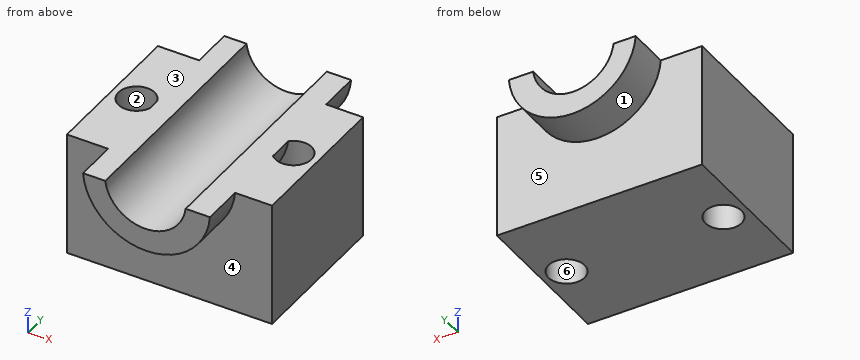
```python
from build123d import *

# Parameters (mm, degrees)
F0_W     = 86.4731967449
F0_H     = 64.1862973571
F1_DEPTH = 52.578
F2_R     = 7.62
F3_DEPTH = 180.34
F5_DEPTH = 49.784
F7_DEPTH = 69.342


with BuildPart() as f1:
    # F0 (on Top) → F1 (new body)
    with BuildSketch(Plane.XY):
        Rectangle(F0_W, F0_H)
    extrude(amount=F1_DEPTH)

    # F2 (on Top) → F3 (cut)
    with BuildSketch(Plane.XY):
        with Locations((33.0765983725, 0)):
            Circle(F2_R)
        with Locations((-33.0765983725, 0)):
            Circle(F2_R)
    extrude(amount=F3_DEPTH, mode=Mode.SUBTRACT)

    # F4 (on Front) → F5 (join, symmetric)
    with BuildSketch(Plane.XZ):
        with BuildLine():
            ThreePointArc((17.383787781, 52.578), (0.4457375035, 37.4617067344), (-16.4923127741, 52.578))
            Line((-16.4923127741, 52.578), (-25.8528143167, 52.578))
            ThreePointArc((-25.8528143167, 52.578), (0.8914759383, 27.7956383617), (27.6357661933, 52.578))
            Line((27.6357661933, 52.578), (17.383787781, 52.578))
        make_face()
    extrude(amount=F5_DEPTH, both=True)

    # F7 (cut): a face of the model
    f7_faces = [f1.faces().sort_by_distance(p)[0] for p in [
        (0.4457375035, 32.0931486785, 46.2197735841),
    ]]
    extrude(f7_faces, amount=-F7_DEPTH, mode=Mode.SUBTRACT)


solid = f1.part
```
The model under review builds one solid part; all positions refer to its coordinate system, in mm. Face numbers are marked on the shaded views. A direction names the side the tool comes from. Give positions to 0.01 mm unless a question says otherwise; leave off trailing zeros. Write each loop counter-clockwise with the first axis right and the second up, starting at its lowest first coordinate (ties: lowest second). Pieces come first, ordered by that corner, then holes. Notation, with made-up numbers: (17, 54.25) -> (59, 54.25) arc R22 ccw to (59, 90.25) -> close; hole circle Ø8 at (78.5, 52.25). An arc over 180 degrees is marked (long way). Put each result on its own line as item: value.
(1) We need section B-B, the plane y = 0. Give the boundary of the cut face in (x, z), and give its area (3 significant figures).
Results are:
outline: (-43.24, 0) -> (-40.7, 0) -> (-40.7, 52.58) -> (-43.24, 52.58) -> close; (-25.85, 52.58) arc R26.82 ccw to (-25.46, 49.6) -> (-25.46, 0) -> (25.46, 0) -> (25.46, 43.85) arc R26.82 ccw to (27.64, 52.58) -> (17.38, 52.58) arc R17.05 cw to (-16.49, 52.58) -> close; (40.7, 0) -> (43.24, 0) -> (43.24, 52.58) -> (40.7, 52.58) -> close
area: 2,570 mm²
(2) We need section C-C, the plane z = 41.5. Give the boundary of the cut face in (x, y), and give its area (3 significant figures).
Results are:
outline: (-43.24, -32.09) -> (-22.5, -32.09) -> (-22.5, -49.78) -> (-10.57, -49.78) -> (-10.57, 49.78) -> (-22.5, 49.78) -> (-22.5, 32.09) -> (-43.24, 32.09) -> close; (11.46, -49.78) -> (24.29, -49.78) -> (24.29, -32.09) -> (43.24, -32.09) -> (43.24, 32.09) -> (24.29, 32.09) -> (24.29, 49.78) -> (11.46, 49.78) -> close; hole circle Ø15.24 at (-33.08, 0); hole circle Ø15.24 at (33.08, 0)
area: 4,650 mm²
(3) Tool access review of the marked faces 4, 5 and 6: name each direction out of +Z, -Z, +X, -X, +Y, -Y from which nothing blocks a thin tool from reaching the whole face with its end or side.
Results are:
face 4: -Z, -Y
face 5: -Z, +Y
face 6: -Z
(4) We need section D-D, the plane y = -29. Give the boundary of the cut face in (x, z), and give its area (3 significant figures).
Results are:
outline: (-43.24, 0) -> (43.24, 0) -> (43.24, 52.58) -> (17.38, 52.58) arc R17.05 cw to (-16.49, 52.58) -> (-43.24, 52.58) -> close
area: 4,160 mm²
(5) We need section A-A, the plane z = 7.5. Give the boundary of the cut face in (x, y), and give its area (3 significant figures).
Results are:
outline: (-43.24, -32.09) -> (43.24, -32.09) -> (43.24, 32.09) -> (-43.24, 32.09) -> close; hole circle Ø15.24 at (-33.08, 0); hole circle Ø15.24 at (33.08, 0)
area: 5,190 mm²
(6) To check wall thickness, follow probe 1 along Y at (x, z) = (-33.5, 32); probe 2 along X at (y, z) = (-6, 23); probe 3 along X at (y, z) = (7, 42.5). State the ranges of each line that lie inside material, in increasing order. Write a range as from..to.
Results are:
probe 1: -32.09..-7.61, 7.61..32.09
probe 2: -43.24..-37.77, -28.38..28.38, 37.77..43.24
probe 3: -43.24..-36.09, -30.07..-11.65, 12.55..30.07, 36.09..43.24
(7) The part is to be moulded in two halves that separate along X. For the marked faces 1, 2 and 3, say which applies: pulls with the +X half, pulls with the -X half, needs draft (parallel to the pull), parting line crosses it, or undercut.
Results are:
face 1: parting line crosses it
face 2: undercut
face 3: needs draft
(8) For pin 1 Ø16 at (x, z) = (16, 22) entering from +Y, flat-tipped, find the tip position at first contact; note if it passes through.
Results are:
pin 1: y = 32.09
